Could you check a few things on this model? Use its own coordinates, in mm. A direction names the side the tool comes from. Give positions to 0.01 mm unless a question says otherwise; leave off trailing zeros. Order: outer loops, then holes, each group sorted by start corner. A loop starts at its lowest first (then second) coordinate and runs counter-clockwise, first axis right, second up.
(1) Imagine slicing it at B-B, the plane z = 14. Write out the boundary of the cut face in (x, y), then the cut area to 3 significant figures.
(2) Imagine slicing it at C-C, the plane x = 39.5. Write out the boundary of the cut face in (y, z), then the cut area to 3 significant figures.
(3) If I drill on probe 1 along Y at (x, z) = (69.5, 55.5); probe 2 along X at (y, z) = (-37, 35.5); probe 3 along X at (y, z) = (-5, 53), over which ranges is the centre line in solid material (lowest first)?
(4) On a 3-axis mill with a long thin cutter (end or side, diameter ignored), from which of +Z, -Z, +X, -X, +Y, -Y can I reach the whole of each face in a straight line? I mean faces 5 (the flat face through (47.283, -47, 32)), 6 (the flat face through (34, -47, 44.916)), 7 (the flat face through (34, -47, 19.516)), 8 (the cylindrical face through (82.231, 12.114, 40.934)). Say none if no direction works.
(5) Imagine slicing it at A-A, the plane y = 0. Write out the boundary of the cut face in (x, z).
(6) Will these pins go through, and if not, where does the flat tip stop? pin 1 (4 mm diameter, centred on y = -2, z = 22, fed in from -X); pin 2 (1 mm diameter, centred on y = -41, z = 10.5, fed in from +X); pin 3 (5 mm diameter, centred on x = 15.5, z = 58.5, fed in from -Y); pin 4 (3.5 mm diameter, centred on y = -49.5, z = 37.5, fed in from +X).
(7) Imagine slicing it at D-D, the plane y = -34. Write out the boundary of the cut face in (x, z), then the cut area to 3 significant figures.
(8) If we mould it in two halves opening along Y, with no side actions, what happens to faces 1 (the flat face through (38, 41.148, 38)), 2 (the flat face through (21.883, -47, 32)), 3 (the flat face through (34, -52.578, 32)), 4 (the cylindrical face through (51.504, 0.558, 37.369))? For each: released by +Y, released by -Y, zero draft, split by the parting line, or undercut.
from build123d import *

# Parameters (mm, degrees)
F0_W     = 76.5958726406
F0_H     = 75.7986828685
F1_DEPTH = 41.148
F3_D     = 25.4
F4_W     = 25.4
F4_H     = 25.4
F5_DEPTH = 11.43
F6_R     = 12.7
F7_DEPTH = 11.43


with BuildPart() as f1:
    # F0 (on Front) → F1 (new body, symmetric)
    with BuildSketch(Plane.XZ):
        with Locations((38.2979363203, 37.8993414342)):
            Rectangle(F0_W, F0_H)
    extrude(amount=F1_DEPTH, both=True)

    # F3 (through all)
    with Locations(Plane.XY.offset(75.7986828685)):
        with Locations((38.8162694871, 0)):
            Hole(F3_D / 2)

    # F4 (on face) → F5 (join)
    with BuildSketch(Plane.XZ.offset(41.148)):
        with Locations((34.5825459808, 32.216026066)):
            Rectangle(F4_W, F4_H)
    extrude(amount=F5_DEPTH)

    # F6 (on face) → F7 (join)
    with BuildSketch(Plane.YZ.offset(76.5958726406)):
        with Locations((0, 37.119705635)):
            Circle(F6_R)
    extrude(amount=F7_DEPTH)


solid = f1.part
Answer block:
1. outline: (0, -41.15) - (76.6, -41.15) - (76.6, 41.15) - (0, 41.15) - close; hole circle Ø25.4 at (38.82, 0)
1. area: 5,800 mm2
2. outline: (-52.58, 19.52) - (-41.15, 19.52) - (-41.15, 0) - (-12.68, 0) - (-12.68, 75.8) - (-41.15, 75.8) - (-41.15, 44.92) - (-52.58, 44.92) - close; (12.68, 0) - (41.15, 0) - (41.15, 75.8) - (12.68, 75.8) - close
2. area: 4,610 mm2
3. probe 1: y = -41.15 to 41.15
3. probe 2: x = 0 to 76.6
3. probe 3: x = 0 to 27.14, 50.49 to 76.6
4. face 5: +Z, -Z, +X, -Y
4. face 6: +Z, +X, -X, -Y
4. face 7: -Z, +X, -X, -Y
4. face 8: +X
5. outline: (0, 0) - (26.12, 0) - (26.12, 75.8) - (0, 75.8) - close; (51.52, 0) - (76.6, 0) - (76.6, 24.42) - (88.03, 24.42) - (88.03, 49.82) - (76.6, 49.82) - (76.6, 75.8) - (51.52, 75.8) - close
6. pin 1: stops at x = 0
6. pin 2: stops at x = 76.6
6. pin 3: stops at y = -41.15
6. pin 4: stops at x = 47.28
7. outline: (0, 0) - (76.6, 0) - (76.6, 75.8) - (0, 75.8) - close
7. area: 5,810 mm2
8. face 1: released by +Y
8. face 2: zero draft
8. face 3: released by -Y
8. face 4: undercut
